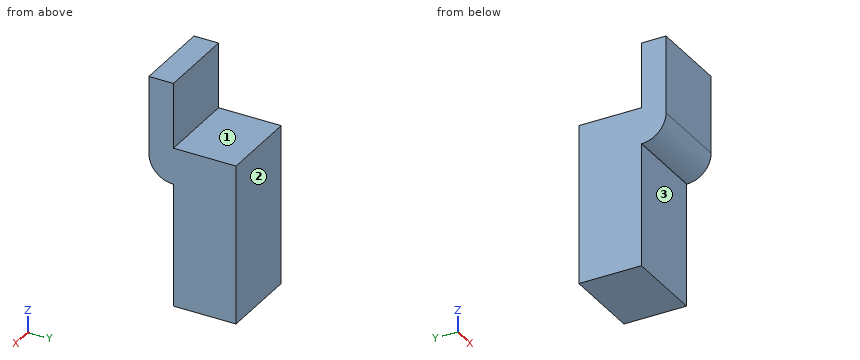
from build123d import *

# Parameters (mm, degrees)
F0_W     = 44.6442011744
F0_H     = 34.9367577583
F1_DEPTH = 88.9
F2_W     = 44.6442011744
F2_H     = 56.7069426179
F3_DEPTH = 13.716
F4_R     = 13.4906253865


with BuildPart() as f1:
    # F0 (on Top) → F1 (new body)
    with BuildSketch(Plane.XY):
        with Locations((33.164284192, 7.5076622888)):
            Rectangle(F0_W, F0_H)
    extrude(amount=F1_DEPTH)

    # F2 (on face) → F3 (join)
    with BuildSketch(Plane.XZ.offset(9.9607165903)):
        with Locations((33.164284192, 96.9944112003)):
            Rectangle(F2_W, F2_H)
    extrude(amount=F3_DEPTH)

    # F4
    f4_edges = [f1.edges().sort_by_distance(p)[0] for p in [
        (33.164284, -23.676717, 68.64094),
    ]]
    fillet(f4_edges, radius=F4_R)


solid = f1.part
For this review, take the finished solid that the model builds, in its own axes (mm). Face numbers are marked on the shaded views. A direction names the side the tool comes from. Round coordinates to 2 decimals unless told otherwise and drop trailing zeros. Loops run counter-clockwise (first coordinate to the right, second up) from the corner with the lowest first, then second, coordinate; pieces in that order, holes last. Notation, with made-up numbers: (-17.5, 15) - (7.5, 15) arc R12 cw to (7.5, 33) - close; hole circle Ø11 at (-6.75, -18.75). An arc over 180 degrees is marked (long way). One line per question, with ' | ' between items.
Q1. For line 1 along Z through (x, y) = (50.5, -10); line 2 along Y through (x, z) = (32.5, 20); line 3 along Y through (x, z) = (22, 89), list the stretches that pass through material, from the lowest coordinate up. Write a range as [from, to].
Taken from the geometry:
line 1: z = [68.64, 125.35] | line 2: y = [-9.96, 24.98] | line 3: y = [-23.68, -9.96]
Q2. Tool access review of the marked faces 1, 2 and 3: name each direction out of +Z, -Z, +X, -X, +Y, -Y from which nothing blocks a thin tool from reaching the whole face with its end or side.
Taken from the geometry:
face 1: +Z, +X, -X, +Y | face 2: +Z, -Z, +X, -X, +Y | face 3: -Z, +X, -X, -Y
Q3. Take a section at C-C (z = 105). Give the boundary of the cut face in (x, y).
Taken from the geometry:
outline: (10.84, -23.68) - (55.49, -23.68) - (55.49, -9.96) - (10.84, -9.96) - close
Q4. For pin 1 (2 mm diameter, centred on x = 44, y = -3, fed in from +Z); pin 2 (11 mm diameter, centred on x = 29, z = 100, fed in from +Y); pin 3 (22.5 mm diameter, centred on x = 38.5, z = 32.5, fed in from -Y), all flat-tipped, find the tip position at first contact; note any pin that passes through.
Taken from the geometry:
pin 1: stops at z = 88.9 | pin 2: stops at y = -9.96 | pin 3: stops at y = -9.96
Q5. Take a section at A-A (x = 45.5). Give the boundary of the cut face in (y, z).
Taken from the geometry:
outline: (-23.68, 82.13) arc R13.49 ccw to (-10.19, 68.64) - (-9.96, 68.64) - (-9.96, 0) - (24.98, 0) - (24.98, 88.9) - (-9.96, 88.9) - (-9.96, 125.35) - (-23.68, 125.35) - close
Q6. Take a section at B-B (y = 10.5). Give the boundary of the cut face in (x, z), and give its area (3 significant figures).
Taken from the geometry:
outline: (10.84, 0) - (55.49, 0) - (55.49, 88.9) - (10.84, 88.9) - close | area: 3,970 mm²
